from build123d import *

# Parameters (mm, degrees)
ESQUISSE1_R             = 25
ESQUISSE1_R_2           = 1
ESQUISSE1_W             = 7.5
ESQUISSE1_H             = 5
BOSS_EXTRU_1_DEPTH      = 5
ESQUISSE2_R             = 21.284112143
ENL_V_MAT_EXTRU_1_DEPTH = 3


with BuildPart() as part:
    # Esquisse1 → Boss.-Extru.1 (new body)
    with BuildSketch(Plane.XY):
        Circle(ESQUISSE1_R)
        with Locations((0, -15)):
            Circle(ESQUISSE1_R_2, mode=Mode.SUBTRACT)
        with Locations((0.05, 0)):
            Rectangle(ESQUISSE1_W, ESQUISSE1_H, mode=Mode.SUBTRACT)
    extrude(amount=BOSS_EXTRU_1_DEPTH)

    # Esquisse2 → Enlèv. mat.-Extru.1 (cut)
    with BuildSketch(Plane.XY.offset(5)):
        Circle(ESQUISSE2_R)
    extrude(amount=-ENL_V_MAT_EXTRU_1_DEPTH, mode=Mode.SUBTRACT)


solid = part.part
Can you work these out from the model? Positions are in its coordinate system, mm. A direction names the side the tool comes from. Coordinates: 2 decimals unless noted, no trailing zeros. Write each loop counter-clockwise with the first axis right and the second up, starting at its lowest first coordinate (ties: lowest second). Pieces come first, ordered by that corner, then holes. Notation, with made-up numbers: (37.25, 58.25) - (60.25, 58.25) arc R28 ccw to (60.25, 85.25) - close; hole circle Ø8 at (-26.75, 76). An arc over 180 degrees is marked (long way). Return JSON: item names as keys, results as strings. Group by question number.
Item 1: If we section it at A-A (x = 0): Write out the boundary of the cut face in (y, z).
Item 2: Which directions (+Z, -Z, +X, -X, +Y, -Y) give clear straight access to the entire face, cutting with the end or side of a thin tool? Please do faces 1 (the face through (0, -5, 0)), 2 (the face through (0, 2.5, 1)).
Item 3: Please list where these lines run through material, in increasing order: probe 1 along Y at (x, z) = (0, 1.5); probe 2 along Y at (x, z) = (0, 3.8); probe 3 along X at (y, z) = (-0.5, 4.35) (3 decimals).
Item 4: We'd pull the mould along Y, two halves only. Please class faces 3 (the face through (23.846, 7.509, 2.465)), 4 (the face through (18.4, 11.2, 5)), 5 (the face through (4, 0, 2)), 6 (the face through (20.3, 6.4, 3.5)): pulls with the +Y half, pulls with the -Y half, needs draft (parallel to the pull), parting line crosses it, or undercut.
Item 5: I'm going to push flat-ended pins straight in: pin 1 Ø2 at (y, z) = (-0.5, 1) entering from +X; pin 2 Ø1.6 at (y, z) = (-1, 1) entering from -X; pin 3 Ø2 at (x, z) = (-0.5, 1) entering from +Y; pin 4 Ø0.6 at (x, z) = (-1.5, 1.5) entering from -Y. Where does each tip first touch, or does it pass through?
Item 6: If we section it at B-B (y = 0): Write out the boundary of the cut face in (x, z), then the cut area to 3 significant figures.
Item 7: If we section it at D-D (y = -11): Write out the boundary of the cut face in (x, z), then the cut area to 3 significant figures.
Item 8: If we section it at C-C (z = 0.8): Write out the boundary of the cut face in (x, y), then the cut area to 3 significant figures.
Return value:
{
 "1": {"outline": "(-25, 0) - (-16, 0) - (-16, 2) - (-21.28, 2) - (-21.28, 5) - (-25, 5) - close; (-14, 0) - (-2.5, 0) - (-2.5, 2) - (-14, 2) - close; (2.5, 0) - (25, 0) - (25, 5) - (21.28, 5) - (21.28, 2) - (2.5, 2) - close"},
 "2": {"face 1": "-Z, +X, -X, +Y, -Y", "face 2": "+Z, -Z"},
 "3": {"probe 1": "y = -25 to -16, -14 to -2.5, 2.5 to 25", "probe 2": "y = -25 to -21.28, 21.28 to 25", "probe 3": "x = -24.995 to -21.278, 21.278 to 24.995"},
 "4": {"face 3": "parting line crosses it", "face 4": "needs draft", "face 5": "undercut", "face 6": "undercut"},
 "5": {"pin 1": "stops at x = 25", "pin 2": "stops at x = -25", "pin 3": "stops at y = 25", "pin 4": "stops at y = -24.97"},
 "6": {"outline": "(-25, 0) - (-3.7, 0) - (-3.7, 2) - (-21.28, 2) - (-21.28, 5) - (-25, 5) - close; (3.8, 0) - (25, 0) - (25, 5) - (21.28, 5) - (21.28, 2) - (3.8, 2) - close", "area": "107 mm^2"},
 "7": {"outline": "(-22.45, 0) - (22.45, 0) - (22.45, 5) - (18.22, 5) - (18.22, 2) - (-18.22, 2) - (-18.22, 5) - (-22.45, 5) - close", "area": "115 mm^2"},
 "8": {"outline": "circle Ø50 at (0, 0); hole (-3.7, -2.5) - (3.8, -2.5) - (3.8, 2.5) - (-3.7, 2.5) - close; hole circle Ø2 at (0, -15)", "area": "1,920 mm^2"}
}
